The model under review builds one solid part; all positions refer to its coordinate system, in mm. Face numbers are marked on the shaded views. A direction names the side the tool comes from. Coordinates: 2 decimals unless noted, no trailing zeros. Order: outer loops, then holes, each group sorted by start corner. A loop starts at its lowest first (then second) coordinate and runs counter-clockwise, first axis right, second up. Notation, with made-up numbers: (25, 80.5) -> (45, 80.5) arc R16 cw to (45, 103.5) -> close; hole circle Ø1 at (-34.75, 70). An arc over 180 degrees is marked (long way). Put each result on its own line as item: value.
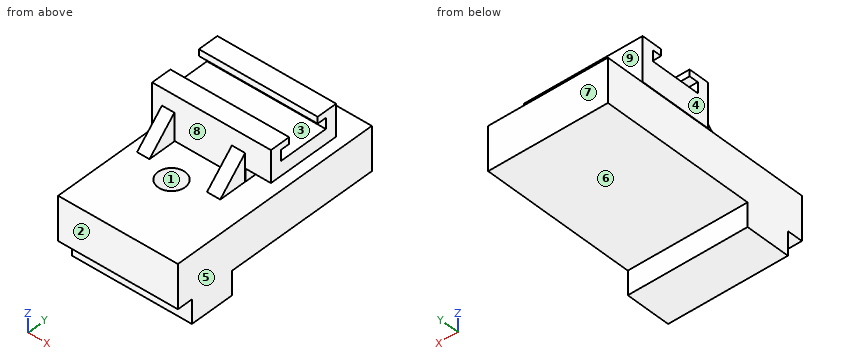
from build123d import *

# Parameters (mm, degrees)
F1_DEPTH    = 84.328
F2_W        = 8.7442607619
F2_H        = 19.8203269392
F2_W_2      = 9.3272216618
F3_DEPTH    = 25.4
F4_T4_DEPTH = 139.3857565506
F4_T9_DEPTH = 139.9687174505
F5_R        = 9.525
F6_DEPTH    = 36.83
F8_DEPTH    = 51.308
F10_DEPTH   = 88.9


# Not quite as in the source:
# - a fillet or chamfer that OpenCascade refuses, or shapes differently, is made with other operations: its cross-section is extruded or revolved along the edge and cut away or added


with BuildPart() as f1:
    # F0 (on Right) → F1 (new body)
    with BuildSketch(Plane.YZ):
        Polygon((78.6539154417, 24.2497121325), (-73.9903064734, 24.2497121325), (-73.9903064734, -6.584421545), (-62.9999262101, -6.584421545), (-62.9999262101, -23.3752859166), (-31.2499262101, -23.3752859166), (-31.2499262101, -6.584421545), (78.6539154417, -6.584421545), align=None)
    extrude(amount=F1_DEPTH)

    # F2 (on Front) → F3 (join)
    with BuildSketch(Plane.XZ):
        with Locations((11.2704045605, 33.9568844065)):
            Rectangle(F2_W, F2_H)
        with Locations((60.8212258667, 33.9568844065)):
            Rectangle(F2_W_2, F2_H)
    extrude(amount=F3_DEPTH)

    # F4: chamfer of 25.4 on 2 edges, made by hand


with BuildPart() as f4_tool2:
    # F4_s3 → F4_t4 (new body)
    with BuildSketch(Plane.YZ.offset(80.9632828358)):
        Polygon((-25.4, 18.4670478761), (0, 43.8670478761), (-25.4, 43.8670478761), align=None)
    extrude(amount=-F4_T4_DEPTH)

    split(bisect_by=Plane.XY.offset(24.2497121325), keep=Keep.TOP)


with BuildPart() as f1_1:
    add(f1.part)

    # F4_t1: cut F4_tool2
    add(f4_tool2.part, mode=Mode.SUBTRACT)


with BuildPart() as f4_tool7:
    # F4_s8 → F4_t9 (new body)
    with BuildSketch(Plane.YZ.offset(130.8055845919)):
        Polygon((-25.4, 18.4670478761), (0, 43.8670478761), (-25.4, 43.8670478761), align=None)
    extrude(amount=-F4_T9_DEPTH)

    split(bisect_by=Plane.XY.offset(24.2497121325), keep=Keep.TOP)


with BuildPart() as f1_2:
    add(f1_1.part)

    # F4_t6: cut F4_tool7
    add(f4_tool7.part, mode=Mode.SUBTRACT)

    # F5 (on Top) → F6 (cut)
    with BuildSketch(Plane.XY):
        with Locations((35.4578830302, -24.3916343898)):
            Circle(F5_R)
    extrude(amount=F6_DEPTH, mode=Mode.SUBTRACT)

    # F7 (on Front) → F8 (join)
    with BuildSketch(Plane.XZ):
        Polygon((65.8567920327, 24.6296729892), (65.8567920327, 33.3739332855), (83.636790514, 33.3739332855), (83.636790514, 55.8175444603), (0, 55.8175444603), (0, 24.6296729892), align=None)
    extrude(amount=-F8_DEPTH)

    # F9 (on Right) → F10 (cut)
    with BuildSketch(Plane.YZ):
        Polygon((36.7869585752, 56.1090186238), (14.3433511257, 56.1090186238), (14.3433511257, 51.153935492), (7.930893451, 51.153935492), (7.930893451, 43.5755737126), (43.1994171752, 43.5755737126), (43.1994171752, 51.153935492), (36.7869585752, 51.153935492), align=None)
    extrude(amount=F10_DEPTH, mode=Mode.SUBTRACT)


solid = f1_2.part
Item 1: For line 1 (Z direction, x = 4.5, y = 9); line 2 (Z direction, x = 11, y = 50); line 3 (Y direction, x = 22.5, z = 51), list the stretches that pass through material, from the lowest coordinate up. Write a range as from..to.
Answers below:
line 1: -6.58..24.25, 24.63..43.58, 51.15..55.82
line 2: -6.58..24.25, 24.63..55.82
line 3: 0..7.93, 43.2..51.31
Item 2: Consider section B-B on x = 76. Write out the cut boundary in (y, z).
Answers below:
outline: (-73.99, -6.58) -> (-63, -6.58) -> (-63, -23.38) -> (-31.25, -23.38) -> (-31.25, -6.58) -> (78.65, -6.58) -> (78.65, 24.25) -> (-73.99, 24.25) -> close; (0, 33.37) -> (51.31, 33.37) -> (51.31, 55.82) -> (36.79, 55.82) -> (36.79, 51.15) -> (43.2, 51.15) -> (43.2, 43.58) -> (7.93, 43.58) -> (7.93, 51.15) -> (14.34, 51.15) -> (14.34, 55.82) -> (0, 55.82) -> close
Item 3: For pin 1 Ø18.5 at (x, z) = (47, -15.5) entering from +Y; pin 2 Ø5 at (x, z) = (74.5, -15) entering from +Y; pin 3 Ø5.5 at (x, y) = (54.5, -71) entering from -Z; pin 4 Ø5 at (x, z) = (45, 53) entering from +Y, all flat-tipped, find the tip position at first contact; note any pin that passes through.
Answers below:
pin 1: y = 78.65
pin 2: y = -31.25
pin 3: z = -6.58
pin 4: y = 51.31
Item 4: Consider section C-C on z = 47.5. Write out the cut boundary in (x, y), and give its area (3 significant figures).
Answers below:
outline: (0, 0) -> (83.64, 0) -> (83.64, 7.93) -> (0, 7.93) -> close; (0, 43.2) -> (83.64, 43.2) -> (83.64, 51.31) -> (0, 51.31) -> close
area: 1,340 mm^2
Item 5: Mouldability with a two-part tool opening along Y and no side actions: class the marked faces 1, 2, 3 and 4 as +Y half, -Y half, draft (parallel to the pull), parting line (faces both ways), or undercut.
Answers below:
face 1: undercut
face 2: -Y half
face 3: undercut
face 4: draft
Item 6: For the marked faces 5, 6, 7, 8 and 9, list the 3-axis set-ups (+Z, -Z, +X, -X, +Y, -Y) from which the entire face can be reached by the end or side of a thin tool; tool diameter is ignored.
Answers below:
face 5: +Z, -Z, +X, +Y, -Y
face 6: -Z, +X, -X, +Y
face 7: +Z, -Z, +X, -X, +Y
face 8: +Z, -Y
face 9: +Z, +X, -X, +Y
Item 7: Consider section D-D on x = 19.5. Write out the cut boundary in (y, z).
Answers below:
outline: (-73.99, -6.58) -> (-63, -6.58) -> (-63, -23.38) -> (-31.25, -23.38) -> (-31.25, -6.58) -> (78.65, -6.58) -> (78.65, 24.25) -> (-73.99, 24.25) -> close; (0, 24.63) -> (51.31, 24.63) -> (51.31, 55.82) -> (36.79, 55.82) -> (36.79, 51.15) -> (43.2, 51.15) -> (43.2, 43.58) -> (7.93, 43.58) -> (7.93, 51.15) -> (14.34, 51.15) -> (14.34, 55.82) -> (0, 55.82) -> close
Item 8: Consider section A-A on y = 25.5. Write out the cut boundary in (x, z).
Answers below:
outline: (0, -6.58) -> (84.33, -6.58) -> (84.33, 24.25) -> (0, 24.25) -> close; (0, 24.63) -> (65.86, 24.63) -> (65.86, 33.37) -> (83.64, 33.37) -> (83.64, 43.58) -> (0, 43.58) -> close
